Can you work these out from the model? Positions are in its coordinate system, mm. Coordinates: 2 decimals unless noted, no trailing zeros. Loops run counter-clockwise (first coordinate to the right, second up) from the corner with the lowest first, then second, coordinate; pieces in that order, holes last. Notation, with made-up numbers: (-28, 17.25) - (0, 17.25) arc R21 ccw to (0, 41.25) - close; hole circle Ø8 at (60.5, 36). An arc over 180 degrees is marked (long way). Put each result on its own line as item: value. Start each with the question number.
from build123d import *

# Parameters (mm, degrees)
F0_R     = 30
F1_DEPTH = 25


with BuildPart() as f1:
    # F0 (on Front) → F1 (new body)
    with BuildSketch(Plane.XZ):
        with BuildLine():
            ThreePointArc((-362.569757, 216.779084), (-355.273719, 196.83206), (-359.21774, 175.961971))
            ThreePointArc((-359.21774, 175.961971), (-339.40005, -211.678071), (0, -400))
            Line((0, -400), (420, -400))
            ThreePointArc((420, -400), (522.212386, -379.905238), (609.21045, -322.61206))
            ThreePointArc((609.21045, -322.61206), (655.448706, -296.833079), (708.368113, -298.271389))
            ThreePointArc((708.368113, -298.271389), (756.702225, -275.904298), (739.970789, -225.342135))
            ThreePointArc((739.970789, -225.342135), (702.734149, -187.712825), (689.925394, -136.346805))
            ThreePointArc((689.925394, -136.346805), (660.297364, -6.885514), (572.529747, 92.788412))
            Line((572.529747, 92.788412), (225.969995, 330.056906))
            ThreePointArc((225.969995, 330.056906), (-33.631094, 398.583679), (-278.079557, 287.526972))
            ThreePointArc((-278.079557, 287.526972), (-296.71916, 277.344579), (-317.943757, 278.139835))
            ThreePointArc((-317.943757, 278.139835), (-362.349443, 263.526868), (-362.569757, 216.779084))
        make_face()
        with BuildLine():
            ThreePointArc((228.652554, -290.891749), (-353.45578, 109.402979), (353.002904, 110.855536))
            ThreePointArc((353.002904, 110.855536), (658.821473, -203.920932), (228.652554, -290.891749))
        make_face(mode=Mode.SUBTRACT)
        with Locations((720, -260)):
            Circle(F0_R, mode=Mode.SUBTRACT)
        with Locations((-330, 240)):
            Circle(F0_R, mode=Mode.SUBTRACT)
        with Locations((400, 150)):
            Circle(F0_R, mode=Mode.SUBTRACT)
    extrude(amount=F1_DEPTH)


solid = f1.part
Q1. Please list where these lines run through material, in increasing order: line 1 along Z through (x, y) = (400, -15.25); line 2 along Z through (x, y) = (-207, -16.75); line 3 along X through (y, z) = (-4, 165.5). Write a range as [from, to].
Q2. I want a section at B-B on z = -260. List the corners of the cut face in (x, y) for me, and give its area (3 significant figures).
Q3. Will these pins go through, and if not, where does the flat tip stop? pin 1 (1 mm diameter, centred on x = 327, y = -7.5, fed in from +Z); pin 2 (5 mm diameter, centred on y = -9.5, z = 223, fed in from -X); pin 3 (8 mm diameter, centred on y = -15.5, z = 214, fed in from -X).
Q4. I want a section at D-D on y = -13. List the corners of the cut face in (x, z) for me, and give its area (3 significant figures).
Q5. We'd pull the mould along Z, two halves only. Please class faces 1 (the cylindrical face through (-357.12, -12.32, 96.78)), 2 (the flat face through (207, -12, -400)), 3 (the cylindrical face through (756.37, -12.32, -276.65)): released by +Z, released by -Z, zero draft, split by the parting line, or undercut.
Q6. I want a section at C-C on x = 400. List the corners of the cut face in (y, z) for me.
Q7. I want a section at A-A on x = -113.5. List the corners of the cut face in (y, z) for me.
Calculated:
1. line 1: [-400, -379.2], [119.2, 120], [180, 210.91]
1. line 2: [-342.27, -306.68], [306.68, 342.27]
1. line 3: [-364.16, -330.92], [330.92, 374.31], [425.69, 466.33]
2. outline: (-303.97, -25) - (-263.25, -25) - (-263.25, 0) - (-303.97, 0) - close; (633.54, -25) - (690, -25) - (690, 0) - (633.54, 0) - close; (750, -25) - (760, -25) - (760, 0) - (750, 0) - close
2. area: 2,680 mm2
3. pin 1: z = 261.23
3. pin 2: x = -367.28
3. pin 3: x = -363.41
4. outline: (-362.57, 216.78) arc R40 cw to (-359.22, 175.96) arc R400 ccw to (0, -400) - (420, -400) arc R270 ccw to (609.21, -322.61) arc R100 cw to (708.37, -298.27) arc R40 ccw to (739.97, -225.34) arc R100 cw to (689.93, -136.35) arc R270 ccw to (572.53, 92.79) - (225.97, 330.06) arc R400 ccw to (-278.08, 287.53) arc R40 cw to (-317.94, 278.14) arc R40 ccw to start; hole circle Ø60 at (-330, 240); hole (228.65, -290.89) arc R250 ccw (long way) to (353, 110.86) arc R370 ccw (long way) to start; hole circle Ø60 at (400, 150); hole circle Ø60 at (720, -260)
4. area: 104,000 mm2
5. face 1: undercut
5. face 2: released by -Z
5. face 3: split by the parting line
6. outline: (-25, -400) - (0, -400) - (0, -379.2) - (-25, -379.2) - close; (-25, 119.2) - (0, 119.2) - (0, 120) - (-25, 120) - close; (-25, 180) - (0, 180) - (0, 210.91) - (-25, 210.91) - close
7. outline: (-25, -383.56) - (0, -383.56) - (0, -352.16) - (-25, -352.16) - close; (-25, 352.16) - (0, 352.16) - (0, 383.56) - (-25, 383.56) - close
